Work out the finished part from the listing and answer in its coordinate system (mm). A direction names the side the tool comes from. Coordinates: 2 decimals unless noted, no trailing zeros. Order: outer loops, then holes, each group sorted by start corner. A loop starts at its lowest first (then second) coordinate and runs counter-clockwise, first axis right, second up. Notation, with made-up numbers: M 72,-16.75 L 115,-16.75 A16 ccw 115,11.25 Z; hole C -30,80 d1. An arc over 180 degrees is marked long. Answer in a Markdown table with one row per item. Add a question column.
Item 1: The part is cut by section A-A (x = 50). Write down the section's boundary in (y, z) (3 decimals), then the cut area to 3 significant figures.
Item 2: Which of the six approach directions +Z, -Z, +X, -X, +Y, -Y give full straight-line access (tool end or side, diameter ignored) to faces 1 (the face through (28, 13, 0)), 2 (the face through (28, 3, -14)), 3 (the face through (26, 0, -14))?
Item 3: The part is cut by section B-B (z = -12.5). Write down the section's boundary in (x, y), then the cut area to 3 significant figures.
Item 4: The part is cut by section D-D (z = -2.5). Write down the section's boundary in (x, y).
Item 5: The part is cut by section C-C (y = 12). Write down the section's boundary in (x, z).
Item 6: The mould has two halves that part along Z. Classify faces 4 (the face through (-3, 11, -15)), 5 (the face through (27, 9, -3.425)), 6 (the face through (26, 11, -31.85)): released by +Z, released by -Z, zero draft, split by the parting line, or undercut.
Item 7: Consider line 1 (Y direction, x = 51.5, z = -3.5); line 2 (Z direction, x = 10, y = 13); line 3 (Y direction, x = 22.5, z = -26.5). Determine where each line is inside the solid, lowest interval first. Write a range as from..to.
Item 8: Flat-ended cylindrical pins translate along their axes: pin 1 Ø1 at (x, z) = (4.5, -7.5) entering from +Y; pin 2 Ø1 at (y, z) = (4.5, -17) entering from +X; pin 3 Ø0.6 at (y, z) = (9.5, -16.5) entering from +X. Find the tip coordinate at first contact, or state that the pin passes through.
Autodesk Inventor part; units mm, degrees
ref_plane "YZ Plane" through (0, 0, 0) normal (1, 0, 0) x (0, 1, 0)
ref_plane "XZ Plane" through (0, 0, 0) normal (0, 1, 0) x (-1, 0, 0)
ref_plane "XY Plane" through (0, 0, 0) normal (0, 0, 1) x (1, 0, 0)
sketch "Sketch1" plane through (0, 0, 0) normal (0, 1, 0) x (-1, 0, 0)
  line L0 (0, 0) -> (0, -28.85)
  line L1 (0, -28.85) -> (-51.6, -28.85)
  line L2 (0, 0) -> (-51.6, 0)
  line L3 (-51.6, 0) -> (-51.6, -28.85)
  line L4 (-54.6, -31.85) -> (3, -31.85)
  line L5 (3, -31.85) -> (3, 3)
  line L6 (3, 3) -> (-54.6, 3)
  line L7 (-54.6, 3) -> (-54.6, -31.85)
  dimension "d0" = 28.85
  dimension "d1" = 51.6
  dimension "d2" = 3
extrude "Extrusion1" add sketch "Sketch1" along normal blind 3 contours L0 L1 L3 L2
extrude "Extrusion2" add sketch "Sketch1" along normal blind 23
sketch "Sketch2" plane through (54.6, 0, 3) normal (1, 0, 0) x (0, 0, -1)
  line L0 (3, 3) -> (3, 23)
  line L1 (3, 23) -> (3, 3)
  line L2 (31.85, 3) -> (31.85, 23)
  line L3 (3, 3) -> (31.85, 3)
  line L4 (31.85, 3) -> (31.85, 23)
  line L5 (31.85, 23) -> (3, 23)
  point P0 (3, 0)
extrude "Extrusion3" cut sketch "Sketch2" against normal blind 23
sketch "Sketch3" plane through (0, 3, -28.85) normal (1, 0, 0) x (0, 0, -1)
  line L0 (0, 0) -> (-28.85, 0)
  line L1 (-14.425, 0) -> (-14.425, 5)
  line L2 (-14.425, 5) -> (-3.425, 5)
  line L3 (-14.425, 5) -> (-25.425, 5)
  line L4 (-25.425, 5) -> (-25.425, 7)
  line L5 (-25.425, 7) -> (-3.425, 7)
  line L6 (-3.425, 7) -> (-3.425, 5)
  point P0 (-28.85, -3)
  dimension "d9" = 5
  dimension "d10" = 11
  dimension "d11" = 11
  dimension "d12" = 2
extrude "Extrusion4" add sketch "Sketch3" along normal blind 54
properties part number "DudukanESP32"
Reply:
| question | item | result |
|---|---|---|
| 1 | outline | M 0,-31.85 L 23,-31.85 L 23,-28.85 L 3,-28.85 L 3,0 L 23,0 L 23,3 L 0,3 Z; M 8,-25.425 L 10,-25.425 L 10,-3.425 L 8,-3.425 Z |
| 1 | area | 269 mm2 |
| 2 | face 1 | +X, +Y |
| 2 | face 2 | +X |
| 2 | face 3 | +Z, -Z, +X, -X, -Y |
| 3 | outline | M -3,0 L 54.6,0 L 54.6,3 L 0,3 L 0,8 L 54,8 L 54,10 L 0,10 L 0,23 L -3,23 Z |
| 3 | area | 341 mm2 |
| 4 | outline | M -3,0 L 54.6,0 L 54.6,3 L 0,3 L 0,23 L -3,23 Z |
| 5 | outline | M -3,-31.85 L 54.6,-31.85 L 54.6,-28.85 L 0,-28.85 L 0,0 L 54.6,0 L 54.6,3 L -3,3 Z |
| 6 | face 4 | zero draft |
| 6 | face 5 | undercut |
| 6 | face 6 | released by -Z |
| 7 | line 1 | y = 0..3, 8..10 |
| 7 | line 2 | z = -31.85..-28.85, 0..3 |
| 7 | line 3 | y = 0..3 |
| 8 | pin 1 | stops at y = 10 |
| 8 | pin 2 | stops at x = 0 |
| 8 | pin 3 | stops at x = 54 |
